Input: dimensioned drawing with shaded views. Units: mm. Origin: part minimum x, y, z. Round coordinates to 2 decimals unless told otherwise and drop trailing zeros. Loops run counter-clockwise (first coordinate to the right, second up) from the corner with the lowest first, then second, coordinate; pieces in that order, holes last. Notation, with made-up numbers: M 33,77 L 89,77 A19 ccw 89,113 Z; hole C -5,87.5 d9. An arc over 180 degrees is marked long. Answer as CSV lines item,"result". Start each with the question number.
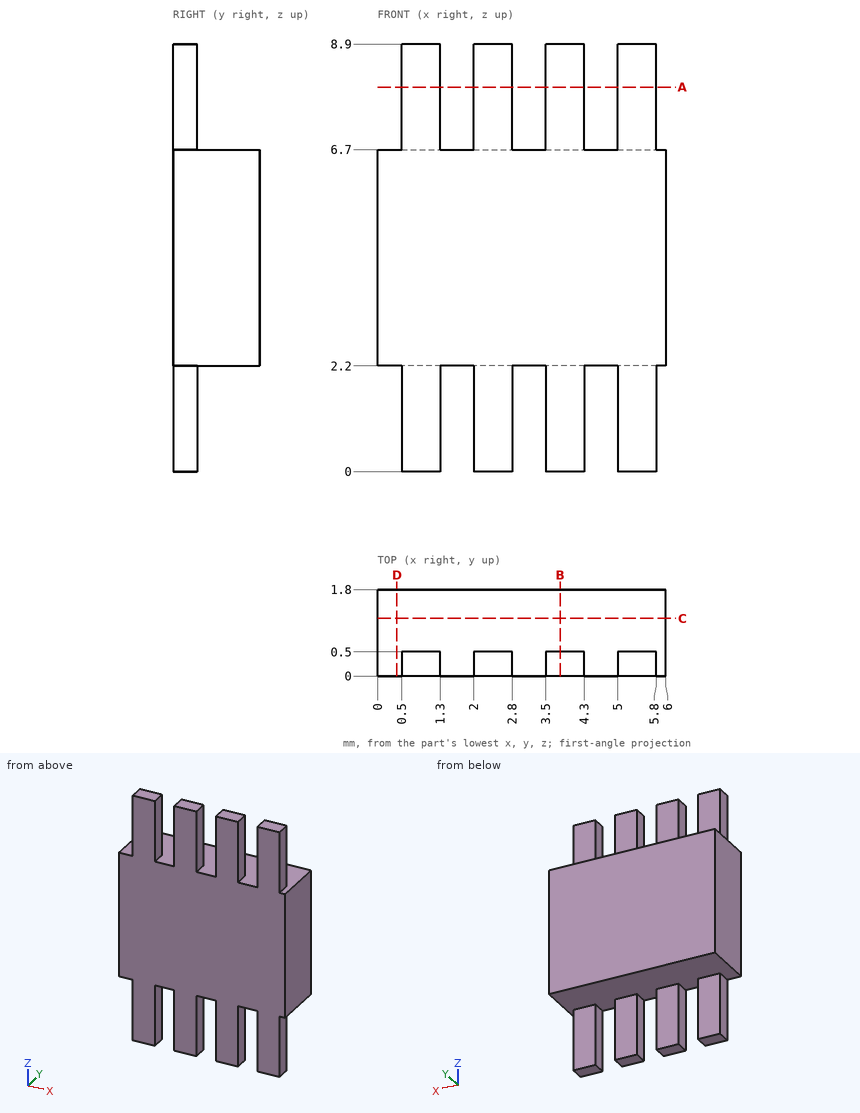
1) Contact query for flat-ended pins moving along their axis: pin 1 Ø0.5 at (x, y) = (2, 1.5) entering from +Z; pin 2 Ø0.9 at (x, z) = (4, 7.5) entering from +Y; pin 3 Ø0.6 at (y, z) = (0.5, 7.5) entering from -X. Output: stop coordinate, or through.
2) Section C-C, the plane y = 1.2. Return loops of the section in (x, z), and give its area (3 significant figures).
3) Section A-A, the plane z = 8. Return loops of the section in (x, y), and give its area (3 significant figures).
4) Ray query, line 1 along X through (y, z) = (0.15, 7.5); line 2 along Y through (x, z) = (2.45, 8.25); line 3 along Z through (x, y) = (4.8, 1.1). Return the intervals inside material, ascending.
5) Section B-B, the plane x = 3.8. Return loops of the section in (y, z), and give its area (3 significant figures).
6) Section D-D, the plane x = 0.4. Return loops of the section in (y, z).
Findings below:
1,pin 1,"z = 6.7"
1,pin 2,"y = 0.5"
1,pin 3,"x = 0.5"
2,outline,"M 0,2.2 L 6,2.2 L 6,6.7 L 0,6.7 Z"
2,area,"27.0 mm²"
3,outline,"M 0.5,0 L 1.3,0 L 1.3,0.5 L 0.5,0.5 Z; M 2,0 L 2.8,0 L 2.8,0.5 L 2,0.5 Z; M 3.5,0 L 4.3,0 L 4.3,0.5 L 3.5,0.5 Z; M 5,0 L 5.8,0 L 5.8,0.5 L 5,0.5 Z"
3,area,"1.60 mm²"
4,line 1,"0.5 to 1.3, 2 to 2.8, 3.5 to 4.3, 5 to 5.8"
4,line 2,"0 to 0.5"
4,line 3,"2.2 to 6.7"
5,outline,"M 0,0 L 0.5,0 L 0.5,2.2 L 1.8,2.2 L 1.8,6.7 L 0.5,6.7 L 0.5,8.9 L 0,8.9 Z"
5,area,"10.3 mm²"
6,outline,"M 0,2.2 L 1.8,2.2 L 1.8,6.7 L 0,6.7 Z"
